from build123d import *

# Parameters (mm, degrees)
EXTRUDE_1_DEPTH     = 3.2
SKETCH_2_R          = 3
CUT_EXTRUDE_1_DEPTH = 5
CHAMFER_1_SIZE      = 0.25


with BuildPart() as part:
    # Эскиз1 → Вытянуть1 (new body)
    with BuildSketch(Plane(origin=(0, 0, 0), x_dir=(1, 0, 0), z_dir=(0, 1, 0))):
        Polygon((-2.886751346, 5), (2.886751346, 5), (5.773502692, 0), (2.886751346, -5), (-2.886751346, -5), (-5.773502692, 0), align=None)
    extrude(amount=EXTRUDE_1_DEPTH)

    # Эскиз2 → Вырез-Вытянуть1 (cut)
    with BuildSketch(Plane(origin=(0, 3.2, 0), x_dir=(-1, 0, 0), z_dir=(0, 1, 0))):
        with Locations(Location((0, 0, 0), (0, 0, 90))):
            Circle(SKETCH_2_R)
    extrude(amount=-CUT_EXTRUDE_1_DEPTH, mode=Mode.SUBTRACT)

    # Эскиз3 → Вырез-Повернуть1 (revolve, cut)
    with BuildSketch(Plane.XY, mode=Mode.PRIVATE) as cut_revolve_1_sk:
        Polygon((-4.5, 3.2), (-6.5, 2.045299462), (-6.5, 3.2), align=None)
        Polygon((-4.5, 0), (-6.5, 1.154700538), (-6.5, 0), align=None)
    revolve(cut_revolve_1_sk.sketch.rotate(Axis((0, 3.2, 0), (0, -1, 0)), 60.000000114), axis=Axis((0, 3.2, 0), (0, -1, 0)), mode=Mode.SUBTRACT)

    # Фаска1
    chamfer_1_edges = [part.edges().sort_by_distance(p)[0] for p in [
        (0, 0, -3),
        (0, 3.2, -3),
    ]]
    chamfer(chamfer_1_edges, length=CHAMFER_1_SIZE)


solid = part.part
CAD build for the part. Positions are in the model's coordinates, mm. Round coordinates to 2 decimals unless told otherwise and drop trailing zeros. Write each loop counter-clockwise with the first axis right and the second up, starting at its lowest first coordinate (ties: lowest second). Pieces come first, ordered by that corner, then holes. Notation, with made-up numbers: M 72.5,24 L 112.5,24 A13 ccw 112.5,40 Z; hole C -23.75,-1 d2. An arc over 180 degrees is marked long. Use a Markdown table: item, result. Add a question column.
1. Pull direction Z, two halves, no side cores. Call faces 1 (the face through (-3, 0, 2)), 2 (the face through (0, 2, -5)), 3 (the face through (0, 2, 5)), 4 (the face through (0.9, 1.62, 2.86)): released by +Z, released by -Z, zero draft, split by the parting line, or undercut.
2. Slice it at A-A on x = 0. Give the cut face in (y, z).
3. Drill centre lines: probe 1 along Z at (x, y) = (1, 2.7); probe 2 along X at (y, z) = (1.9, -0.5); probe 3 along X at (y, z) = (0.9, -2). Where is each one in solid material? Low to high.
4. Slice it at B-B on y = 2. Give the cut face in (x, z).
Reply:
| question | item | result |
|---|---|---|
| 1 | face 1 | zero draft |
| 1 | face 2 | released by -Z |
| 1 | face 3 | released by +Z |
| 1 | face 4 | undercut |
| 2 | outline | M 0,-4.5 L 0.29,-5 L 2.91,-5 L 3.2,-4.5 L 3.2,-3.25 L 2.95,-3 L 0.25,-3 L 0,-3.25 Z; M 0,3.25 L 0.25,3 L 2.95,3 L 3.2,3.25 L 3.2,4.5 L 2.91,5 L 0.29,5 L 0,4.5 Z |
| 3 | probe 1 | z = -5 to -2.83, 2.83 to 5 |
| 3 | probe 2 | x = -5.48 to -2.96, 2.96 to 5.48 |
| 3 | probe 3 | x = -4.62 to -2.24, 2.24 to 4.62 |
| 4 | outline | M -5.77,0 L -2.89,-5 L 2.89,-5 L 5.77,0 L 2.89,5 L -2.89,5 Z; hole C 0,0 d6 |
